from build123d import *

# Parameters (mm, degrees)
EXTRUDE_1_DEPTH = 1


with BuildPart() as part:
    # 草图1 → 凸台-拉伸1 (new body)
    with BuildSketch(Plane.XY):
        with BuildLine():
            Line((13.756161337, -11.589316843), (13.755737728, -11.576233912))
            ThreePointArc((13.755737728, -11.576233912), (16.705777817, -8.371391827), (20.787340615, -6.8500127))
            Line((20.787340615, -6.8500127), (20.787340615, 6.838712609))
            ThreePointArc((20.787340615, 6.838712609), (16.726466447, 8.343658429), (13.805099755, 11.540716072))
            Line((13.805099755, 11.540716072), (13.780842765, 11.560323903))
            Line((13.780842765, 11.560323903), (13.779097734, 11.562037241))
            ThreePointArc((13.779097734, 11.562037241), (-17.987329683, 0.017820318), (13.756161337, -11.589316843))
        make_face()
        with BuildLine():
            Line((-7.815615951, 3.00000508), (0, 3.00000508))
            ThreePointArc((0, 3.00000508), (3.000005067, 1.3e-08), (0, -3.000005054))
            Line((0, -3.000005054), (-7.815615951, -3.000005054))
            ThreePointArc((-7.815615951, -3.000005054), (-10.816019825, 1.3e-08), (-7.815615951, 3.00000508))
        make_face(mode=Mode.SUBTRACT)
    extrude(amount=EXTRUDE_1_DEPTH)


solid = part.part
Geometry: final body of the model. Coordinates: model frame, mm. A direction names the side the tool comes from. Give positions to 0.01 mm unless a question says otherwise; leave off trailing zeros. Write each loop counter-clockwise with the first axis right and the second up, starting at its lowest first coordinate (ties: lowest second). Pieces come first, ordered by that corner, then holes. Notation, with made-up numbers: (-26.75, 70) -> (25.25, 70) arc R21 ccw to (25.25, 96) -> close; hole circle Ø10 at (26, 65). An arc over 180 degrees is marked (long way). Answer as a JSON object with one key per item and string values.
1. Cut plane D-D on x = 5. Output: boundary loops of the cut face in (y, z).
Ans:
{"outline": "(-17.28, 0) -> (17.28, 0) -> (17.28, 1) -> (-17.28, 1) -> close"}
2. Contact query for a flat-ended pin moving along its axis: pin 1 (0.5 mm diameter, centred on x = -2, z = 0.5, fed in from -Y). Output: stop coordinate, or through.
Ans:
{"pin 1": "stops at y = -17.9"}
3. Cut plane B-B on y = 0. Output: boundary loops of the cut face in (x, z).
Ans:
{"outline": "(-17.99, 0) -> (-10.82, 0) -> (-10.82, 1) -> (-17.99, 1) -> close; (3, 0) -> (20.79, 0) -> (20.79, 1) -> (3, 1) -> close"}
4. Cut plane A-A on x = -9. Output: boundary loops of the cut face in (y, z).
Ans:
{"outline": "(-15.57, 0) -> (-2.76, 0) -> (-2.76, 1) -> (-15.57, 1) -> close; (2.76, 0) -> (15.57, 0) -> (15.57, 1) -> (2.76, 1) -> close"}
5. Ray query, probe 1 along X at (y, z) = (-1.5, 0.7); probe 2 along Y at (x, z) = (-2, 0.75); probe 3 along Y at (x, z) = (2.5, 0.7). Return the intervals inside material, ascending. Write a range as from..to.
Ans:
{"probe 1": "x = -17.92..-10.41, 2.6..20.79", "probe 2": "y = -17.88..-3, 3..17.88", "probe 3": "y = -17.81..-1.66, 1.66..17.81"}
6. Access query for faces 1 (the flat face through (-3.9, -3, 0.5)), 2 (the flat face through (20.787, -0.1, 0.5)). Directions: +Z, -Z, +X, -X, +Y, -Y. A direction counts if a zero-diameter tool reaches every point of the face in a straight line with its end or side. Return the directions, or none.
Ans:
{"face 1": "+Z, -Z", "face 2": "+Z, -Z, +X, +Y, -Y"}
7. Mould query, pull axis X, two halves, no side actions, for faces 3 (the cylindrical face through (16.78, 8.31, 0.49)), 4 (the cylindrical face through (3, 0.1, 0.5)), 5 (the flat face through (1, -4, 1)). Classes: pulls with the +X half, pulls with the -X half, needs draft (parallel to the pull), parting line crosses it, or undercut.
Ans:
{"face 3": "pulls with the +X half", "face 4": "undercut", "face 5": "needs draft"}
